Autodesk Inventor part; units mm, degrees
ref_plane "YZ Plane" through (0, 0, 0) normal (1, 0, 0) x (0, 1, 0)
ref_plane "XZ Plane" through (0, 0, 0) normal (0, 1, 0) x (-1, 0, 0)
ref_plane "XY Plane" through (0, 0, 0) normal (0, 0, 1) x (1, 0, 0)
sketch "Sketch1" plane through (0, 0, 0) normal (0, 0, 1) x (1, 0, 0)
  circle A0 centre (0, 0) radius 5
  circle A1 centre (0, 0) radius 8
  dimension "d0" = 10
  dimension "d1" = 16
extrude "Extrusion1" add sketch "Sketch1" along normal blind 4
thread "Thread1"
chamfer "Chamfer1" distance 0.4 angle 45 1 edges at (-5, 0, 4)
chamfer "Chamfer2" distance 0.4 angle 45 1 edges at (-5, 0, 0)
properties part number "nakretka-GM"
Read the model definition and answer for the solid it produces. Units are mm, in the model's axes. Give positions to 0.01 mm unless a question says otherwise; leave off trailing zeros. Write each loop counter-clockwise with the first axis right and the second up, starting at its lowest first coordinate (ties: lowest second). Pieces come first, ordered by that corner, then holes. Notation, with made-up numbers: (75, 46) - (117, 46) arc R19 ccw to (117, 82) - close; hole circle Ø10 at (-40, 76.25). An arc over 180 degrees is marked (long way). Return JSON: item names as keys, results as strings.
Q1. Given P1, Ø8, axis at x = 0, y = 0, coming from the -Z side; P2, Ø1, axis at x = 3.5, z = 3, coming from the -Y side; P3, Ø8, axis at x = 4.5, y = -2, coming from the -Z side, each flat-ended and moving along its own axis, determine where each tip first touches the part or whether it passes through.
Reply:
{"P1": "through", "P2": "y = -7.42", "P3": "z = 0"}
Q2. A cutting plane is placed at A-A, the plane x = 0. Determine the outline of the cut face in (y, z), and give its area (3 significant figures).
Reply:
{"outline": "(-8, 0) - (-5.4, 0) - (-5, 0.4) - (-5, 3.6) - (-5.4, 4) - (-8, 4) - close; (5, 0.4) - (5.4, 0) - (8, 0) - (8, 4) - (5.4, 4) - (5, 3.6) - close", "area": "23.7 mm²"}
Q3. For a pull along X with two mould halves and no side action, classify faces 1 (the face through (5.22, 1.89, 0)), 2 (the face through (-1.08, 4.88, 1.98)), 3 (the face through (-1.73, 7.81, 1.97)) as released by +X, released by -X, zero draft, split by the parting line, or undercut.
Reply:
{"face 1": "zero draft", "face 2": "undercut", "face 3": "split by the parting line"}
Q4. Consider line 1 along Y through (x, z) = (0, 1.1); line 2 along Y through (x, z) = (-4.5, 3.05); line 3 along X through (y, z) = (-1.25, 0.85). Determine where each line is inside the solid, lowest interval first. Write a range as [from, to].
Reply:
{"line 1": "[-8, -5], [5, 8]", "line 2": "[-6.61, -2.18], [2.18, 6.61]", "line 3": "[-7.9, -4.84], [4.84, 7.9]"}
Q5. A cutting plane is placed at D-D, the plane x = 5.75. Determine the outline of the cut face in (y, z), and give its area (3 significant figures).
Reply:
{"outline": "(-5.56, 0) - (5.56, 0) - (5.56, 4) - (-5.56, 4) - close", "area": "44.5 mm²"}
Q6. A cutting plane is placed at C-C, the plane z = 1.5. Determine the outline of the cut face in (x, y), and give its area (3 significant figures).
Reply:
{"outline": "circle Ø16 at (0, 0); hole circle Ø10 at (0, 0)", "area": "123 mm²"}
